Check sheet for the modelled part. Datum: model origin and axes. Units: mm. Face numbers are marked on the shaded views. A direction names the side the tool comes from. Coordinates: 2 decimals unless noted, no trailing zeros. Loops run counter-clockwise (first coordinate to the right, second up) from the corner with the lowest first, then second, coordinate; pieces in that order, holes last. Notation, with made-up numbers: (84, 74.5) - (140, 74.5) arc R21 ccw to (140, 104.5) - close; hole circle Ø10 at (18.5, -24.75). An arc over 180 degrees is marked (long way). Use a Markdown table: item, result. Add a question column.
1) Sectioned sample at A-A, the plane x = 0. Enter the section's corners in (y, z).
2) Sectioned sample at C-C, the plane x = -61.5. Enter the section's corners in (y, z).
3) Sectioned sample at B-B, the plane y = 62.5. Enter the section's corners in (x, z).
4) Tool access check on the marked faces 1 and 2. Record the directions out of +Z, -Z, +X, -X, +Y, -Y that give a thin tool (end or side, any length) a straight path to the whole face; none if there is none.
5) Draft check along Y on the marked faces 3, 4, 5 and 6. Enter one of: pulls with the +Y half, pulls with the -Y half, needs draft (parallel to the pull), parting line crosses it, or undercut.
6) Thickness scan on line 1 (Y direction, x = -38, z = 6.5); line 2 (Z direction, x = 25, y = -36); line 3 (Y direction, x = 1.5, z = 61.5). Record the ranges inside material, lowest first.
7) Go/stop test with flat-tipped pins: P1, Ø2, axis at x = -34.5, y = 22.5, coming from the +Z side; P2, Ø4, axis at x = -11.31, y = 11.31, coming from the +Z side; P3, Ø8, axis at x = 58, z = 8, coming from the -Y side. Record where each tip stops, or that it passes through.
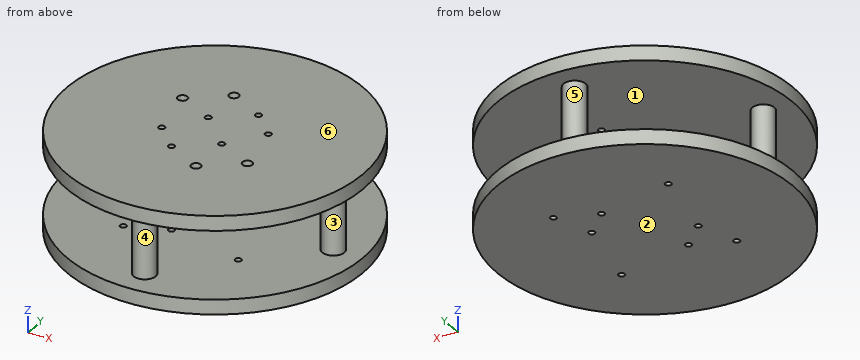
from build123d import *

# Parameters (mm, degrees)
SKETCH_1_R               = 100
EXTRUDE_1_DEPTH          = 10
SKETCH_12_R              = 7.5
EXTRUDE_3_DEPTH          = 46
SKETCH_14_R              = 100
EXTRUDE_4_DEPTH          = 10
SKETCH_15_R              = 2.1
CUT_EXTRUDE_7_DEPTH      = 10
SKETCH_15_3_R            = 2.1
CUT_EXTRUDE_8_DEPTH      = 157.064089399
SKETCH_18_R              = 3.3
CUT_EXTRUDE_9_DEPTH      = 5
HOLE_WIZARD_M5_1_D       = 4.2
HOLE_WIZARD_M5_1_DEPTH   = 10
PATTERN_CIRCULAR_1_COUNT = 4


with BuildPart() as part:
    # 草图1 → 凸台-拉伸1 (new body)
    with BuildSketch(Plane.XY):
        Circle(SKETCH_1_R)
    extrude(amount=EXTRUDE_1_DEPTH)

    # 草图12 → 凸台-拉伸3 (add)
    with BuildSketch(Plane.XY.offset(10)):
        with Locations((-80, 0)):
            Circle(SKETCH_12_R)
        with Locations((0, 80)):
            Circle(SKETCH_12_R)
        with Locations((80, 0)):
            Circle(SKETCH_12_R)
        with Locations((0, -80)):
            Circle(SKETCH_12_R)
    extrude(amount=EXTRUDE_3_DEPTH)

    # 草图14 → 凸台-拉伸4 (add)
    with BuildSketch(Plane.XY.offset(56)):
        Circle(SKETCH_14_R)
    extrude(amount=EXTRUDE_4_DEPTH)

    # 草图15 → 切除-拉伸7 (cut)
    with BuildSketch(Plane.XY.offset(66)):
        with Locations((-11.313708499, 11.313708499)):
            Circle(SKETCH_15_R)
        with Locations((11.313708499, -11.313708499)):
            Circle(SKETCH_15_R)
    extrude(amount=-CUT_EXTRUDE_7_DEPTH, mode=Mode.SUBTRACT)

    # 草图15<3> → 切除-拉伸8 (cut, through all)
    with BuildSketch(Plane.XY.offset(66)):
        with Locations((12.402652942, 28.609540367)):
            Circle(SKETCH_15_3_R)
        with Locations((28.609540367, 12.402652942)):
            Circle(SKETCH_15_3_R)
        with Locations((-12.402652942, -28.609540367)):
            Circle(SKETCH_15_3_R)
        with Locations((-28.609540367, -12.402652942)):
            Circle(SKETCH_15_3_R)
    extrude(amount=-CUT_EXTRUDE_8_DEPTH, mode=Mode.SUBTRACT)

    # 草图18 → 切除-拉伸9 (cut)
    with BuildSketch(Plane.XY.offset(66)):
        with Locations((-11.601229272, 41.114613939)):
            Circle(SKETCH_18_R)
        with Locations((-35.774918891, 23.348558378)):
            Circle(SKETCH_18_R)
        with Locations((11.601229272, -41.114613939)):
            Circle(SKETCH_18_R)
        with Locations((35.774918891, -23.348558378)):
            Circle(SKETCH_18_R)
    extrude(amount=-CUT_EXTRUDE_9_DEPTH, mode=Mode.SUBTRACT)

    # M5 螺纹孔1
    with Locations(Plane(origin=(-38.890872965, 38.890872965, 10), x_dir=(1, 0, 0), z_dir=(0, 0, 1))):
        with Locations((0, 0)):
            hole_wizard_m5_1 = Hole(HOLE_WIZARD_M5_1_D / 2, depth=HOLE_WIZARD_M5_1_DEPTH)

    # 阵列(圆周)1: M5 螺纹孔1 ×4 about axis
    pattern_circular_1_axis = Axis((0, 0, 0), (0, 0, 1))
    for i in range(1, PATTERN_CIRCULAR_1_COUNT):
        add(hole_wizard_m5_1.rotate(pattern_circular_1_axis, i * 360 / PATTERN_CIRCULAR_1_COUNT), mode=Mode.SUBTRACT)


solid = part.part
Solved:
| question | item | result |
|---|---|---|
| 1 | outline | (-100, 0) - (100, 0) - (100, 10) - (87.5, 10) - (87.5, 56) - (100, 56) - (100, 66) - (-100, 66) - (-100, 56) - (-87.5, 56) - (-87.5, 10) - (-100, 10) - close; hole (-72.5, 10) - (72.5, 10) - (72.5, 56) - (-72.5, 56) - close |
| 2 | outline | (-78.85, 0) - (78.85, 0) - (78.85, 10) - (-78.85, 10) - close; (-78.85, 56) - (78.85, 56) - (78.85, 66) - (-78.85, 66) - close |
| 3 | outline | (-78.06, 0) - (78.06, 0) - (78.06, 10) - (-78.06, 10) - close; (-78.06, 56) - (78.06, 56) - (78.06, 66) - (-78.06, 66) - close |
| 4 | face 1 | none |
| 4 | face 2 | -Z, +X, -X, +Y, -Y |
| 5 | face 3 | parting line crosses it |
| 5 | face 4 | undercut |
| 5 | face 5 | undercut |
| 5 | face 6 | needs draft |
| 6 | line 1 | y = -92.5 to -40.79, -36.99 to 36.99, 40.79 to 92.5 |
| 6 | line 2 | z = 0 to 10, 56 to 66 |
| 6 | line 3 | y = -99.99 to 99.99 |
| 7 | P1 | stops at z = 61 |
| 7 | P2 | stops at z = 10 |
| 7 | P3 | stops at y = -84.17 |
